The model under review builds one solid part; all positions refer to its coordinate system, in mm. A direction names the side the tool comes from. Round coordinates to 2 decimals unless told otherwise and drop trailing zeros. Loops run counter-clockwise (first coordinate to the right, second up) from the corner with the lowest first, then second, coordinate; pieces in that order, holes last. Notation, with made-up numbers: (-38, 45.5) -> (-7, 45.5) arc R20 ccw to (-7, 72.5) -> close; hole circle Ø3 at (-34, 77). An arc over 180 degrees is marked (long way). Return JSON: item names as keys, results as strings. Group by question number.
```python
from build123d import *

# Parameters (mm, degrees)
F1_DEPTH = 127
F2_DEPTH = 25.4
F0_R     = 50.8
F3_DEPTH = 50.8


with BuildPart() as f1:
    # F0 (on Front) → F1 (new body)
    with BuildSketch(Plane.XZ):
        Polygon((254, 0), (0, 0), (0, -63.5), (63.5, -63.5), (25.4, -25.4), (228.6, -25.4), (190.5, -63.5), (254, -63.5), align=None)
    extrude(amount=F1_DEPTH)

    # F0 (on Front) → F2 (join)
    with BuildSketch(Plane.XZ):
        with BuildLine():
            Line((43.266761, 121.30561), (0, 0))
            Line((0, 0), (254, 0))
            Line((254, 0), (210.733239, 121.30561))
            ThreePointArc((210.733239, 121.30561), (214.598787, 106.59462), (215.9, 91.44))
            ThreePointArc((215.9, 91.44), (111.84538, 3.841213), (43.266761, 121.30561))
        make_face()
    extrude(amount=F2_DEPTH)

    # F0 (on Front) → F3 (join)
    with BuildSketch(Plane.XZ):
        with BuildLine():
            ThreePointArc((210.733239, 121.30561), (127, 180.34), (43.266761, 121.30561))
            ThreePointArc((43.266761, 121.30561), (111.84538, 3.841213), (215.9, 91.44))
            ThreePointArc((215.9, 91.44), (214.598787, 106.59462), (210.733239, 121.30561))
        make_face()
        with Locations((127, 91.44)):
            Circle(F0_R, mode=Mode.SUBTRACT)
    extrude(amount=F3_DEPTH)


solid = f1.part
```
1. We need section D-D, the plane x = 198. Write out the cut boundary in (y, z).
2. We need section C-C, the plane y = -106.5. Write out the cut boundary in (x, z), then the cut area to 3 significant figures.
3. We need section A-A, the plane y = -32. Write out the cut boundary in (x, z).
4. We need section B-B, the plane x = 127. Write out the cut boundary in (y, z).
5. Tool access review of faces 4 (the face through (210, -63, -44)), 5 (the face through (129, -75, 0)), 6 (the face through (232.67, -12.52, 59.8)), 7 (the face through (135.8, -25.4, 2.5)): name each direction out of +Z, -Z, +X, -X, +Y, -Y from which nothing blocks a thin tool from reaching the whole face with its end or side.
6. Draft analysis for pull direction Z (two halves, no side actions). For faces 1 (the face through (165, -50.8, 53)), 2 (the face through (31, -63, -63.5)), 3 (the face through (45, -63, -45)), state which applies: pulls with the +Z half, pulls with the -Z half, needs draft (parallel to the pull), parting line crosses it, or undercut.
7. For P1, Ø10, axis at x = 181.5, y = -17, coming from the -Z side; P2, Ø3, axis at x = 34.5, y = -27.5, coming from the +Z side; P3, Ø12, axis at x = 60, z = 21, coming from the -Y side, all flat-tipped, find the tip position at first contact; note any pin that passes through.
8. Wall thickness on line 1 (X direction, y = -40, z = 91); line 2 (Z direction, x = 112, y = -46); line 3 (Y direction, x = 135.5, z = 160.5): over which ranges is each line inside the solid? List them lowest first.
Check sheet entries:
{
 "1": {"outline": "(-127, -63.5) -> (0, -63.5) -> (0, -56) -> (-127, -56) -> close; (-127, -25.4) -> (0, -25.4) -> (0, 144.94) -> (-50.8, 144.94) -> (-50.8, 37.94) -> (-25.4, 37.94) -> (-25.4, 0) -> (-127, 0) -> close"},
 "2": {"outline": "(0, -63.5) -> (63.5, -63.5) -> (25.4, -25.4) -> (228.6, -25.4) -> (190.5, -63.5) -> (254, -63.5) -> (254, 0) -> (0, 0) -> close", "area": "9,840 mm²"},
 "3": {"outline": "(0, -63.5) -> (63.5, -63.5) -> (25.4, -25.4) -> (228.6, -25.4) -> (190.5, -63.5) -> (254, -63.5) -> (254, 0) -> (0, 0) -> close; (210.73, 121.31) arc R88.9 ccw (long way) to (215.9, 91.44) arc R88.9 ccw to start; hole circle Ø101.6 at (127, 91.44)"},
 "4": {"outline": "(-127, -25.4) -> (0, -25.4) -> (0, 40.64) -> (-50.8, 40.64) -> (-50.8, 2.54) -> (-25.4, 2.54) -> (-25.4, 0) -> (-127, 0) -> close; (-50.8, 142.24) -> (0, 142.24) -> (0, 180.34) -> (-50.8, 180.34) -> close"},
 "5": {"face 4": "+Y, -Y", "face 5": "+X, -X, -Y", "face 6": "+Z, +X, +Y, -Y", "face 7": "-Y"},
 "6": {"face 1": "needs draft", "face 2": "pulls with the -Z half", "face 3": "undercut"},
 "7": {"P1": "stops at z = -25.4", "P2": "stops at z = 0", "P3": "stops at y = -25.4"},
 "8": {"line 1": "x = 38.1 to 76.2, 177.8 to 215.9", "line 2": "z = -25.4 to 0, 3.81 to 42.91, 139.97 to 179.07", "line 3": "y = -50.8 to 0"}
}
